```python
from build123d import *

# Parameters (mm, degrees)
EXTRUDE_THIN1_DEPTH = 50
SKETCH4_R           = 2.5
CUT_EXTRUDE3_DEPTH  = 206


with BuildPart() as part:
    # Sketch3 → Extrude-Thin1 (new body)
    with BuildSketch(Plane(origin=(0, 0, 0), x_dir=(1, 0, 0), z_dir=(0, 1, 0))):
        Polygon((-1.25, -2.165063509), (71.112159322, -43.943375673), (71.112159322, -110), (-123.887840678, -110), (-123.887840678, -55), (-81.387840678, -55), (-81.387840678, -50), (-128.887840678, -50), (-128.887840678, -115), (76.112159322, -115), (76.112159322, -41.056624327), (1.25, 2.165063509), align=None)
    extrude(amount=EXTRUDE_THIN1_DEPTH)

    # Sketch4 → Cut-Extrude3 (cut, through all)
    with BuildSketch(Plane(origin=(76.112159322, 0, 0), x_dir=(0, 0, -1), z_dir=(1, 0, 0))):
        with Locations((-80.909677613, 24.451666954)):
            Circle(SKETCH4_R)
    extrude(amount=-CUT_EXTRUDE3_DEPTH, mode=Mode.SUBTRACT)


solid = part.part
```
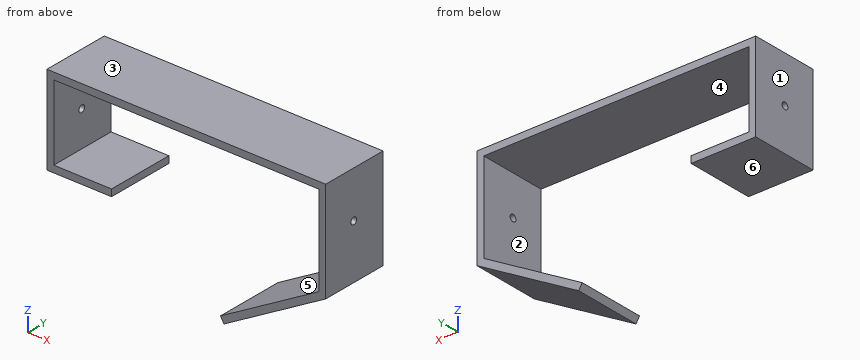
Verification items for the finished model (mm, model axes). Face numbers are marked on the shaded views. A direction names the side the tool comes from. Round coordinates to 2 decimals unless told otherwise and drop trailing zeros. Order: outer loops, then holes, each group sorted by start corner. A loop starts at its lowest first (then second) coordinate and runs counter-clockwise, first axis right, second up.
1) Cross-section at C-C, the plane y = 46. Record the cut outline in (x, z).
Geometry says:
outline: (-128.89, 50) - (-81.39, 50) - (-81.39, 55) - (-123.89, 55) - (-123.89, 110) - (71.11, 110) - (71.11, 43.94) - (-1.25, 2.17) - (1.25, -2.17) - (76.11, 41.06) - (76.11, 115) - (-128.89, 115) - close
2) Depth check by flat-ended pin: pin 1 (3 mm diameter, centred on x = -48.5, y = 8.5, fed in from -Z); pin 2 (2 mm diameter, centred on y = 19.5, z = 18, fed in from -X); pin 3 (1.5 mm diameter, centred on x = 35, y = 39, fed in from -Z). Enter the tip coordinate at first touch or a pass-through.
Geometry says:
pin 1: stops at z = 110
pin 2: stops at x = 24.44
pin 3: stops at z = 16.89
3) Material ranges on line 1 (Z direction, x = -85, y = 33); line 2 (X direction, y = 32.5, z = 100.5); line 3 (Z direction, x = -44.5, y = 5.5), recorded low to high.
Geometry says:
line 1: z = 50 to 55, 110 to 115
line 2: x = -128.89 to -123.89, 71.11 to 76.11
line 3: z = 110 to 115
4) Cross-section at D-D, the plane x = -44.5. Record the cut outline in (y, z).
Geometry says:
outline: (0, 110) - (50, 110) - (50, 115) - (0, 115) - close
5) Cross-section at A-A, the plane x = -96. Record the cut outline in (y, z).
Geometry says:
outline: (0, 50) - (50, 50) - (50, 55) - (0, 55) - close; (0, 110) - (50, 110) - (50, 115) - (0, 115) - close
6) Cross-section at B-B, the plane z = 101.5. Record the cut outline in (x, y).
Geometry says:
outline: (-128.89, 0) - (-123.89, 0) - (-123.89, 50) - (-128.89, 50) - close; (71.11, 0) - (76.11, 0) - (76.11, 50) - (71.11, 50) - close
7) Tool access check on the marked faces 4, 5 and 6. Record the directions out of +Z, -Z, +X, -X, +Y, -Y that give a thin tool (end or side, any length) a straight path to the whole face; none if there is none.
Geometry says:
face 4: +Y, -Y
face 5: -X, +Y, -Y
face 6: -Z, -X, +Y, -Y
8) Draft check along Z on the marked faces 1, 2 and 3. Enter one of: +Z half, -Z half, draft (parallel to the pull), parting line (faces both ways), or undercut.
Geometry says:
face 1: draft
face 2: undercut
face 3: +Z half
